Geometry: final body of the model. Coordinates: model frame, mm. A direction names the side the tool comes from. Give positions to 0.01 mm unless a question says otherwise; leave off trailing zeros. Write each loop counter-clockwise with the first axis right and the second up, starting at its lowest first coordinate (ties: lowest second). Pieces come first, ordered by that corner, then holes. Notation, with made-up numbers: (42.25, 73) -> (65.25, 73) arc R9 cw to (65.25, 87) -> close; hole circle Ø3 at (24.25, 80). An arc over 180 degrees is marked (long way). Use CSV: the item, a comma, the result in double quotes. Start each with the question number.
1) Draft query along Y for faces 1 (the face through (88.026, -49.484, -7.92)), 2 (the face through (80, -47, -1.73)), 3 (the face through (5.595, 0.246, -2.268)). Return one class per face: pulls with the +Y half, pulls with the -Y half, needs draft (parallel to the pull), parting line crosses it, or undercut.
2) Section D-D (x = 95.5). Output: boundary loops of the cut face in (y, z), plus the area to 3 significant figures.
3) Section B-B (y = -16.5). Output: boundary loops of the cut face in (x, z).
4) Contact query for flat-ended pins moving along their axis: P1, Ø1.7, axis at x = 47.5, z = -8, coming from the -Y side; P2, Ø0.9, axis at x = 127.5, z = -0.5, coming from the +Y side; P3, Ø0.6, axis at x = 43.5, z = -7.5, coming from the +Y side; P4, Ø4.5, axis at x = 0, y = 0, coming from the +Z side. Output: stop coordinate, or through.
5) Set-up query: faces 4 (the face through (135.69, -104.06, -7.95)), 5 (the face through (134.696, -103.751, -2.716)), 6 (the face through (9, 0, -4)), 7 (the face through (3, -1, -4.6)). Return all of +Z, -Z, +X, -X, +Y, -Y with unobstructed straight access to the full face (end or side cutting, diameter ignored); none if empty.
6) Section A-A (x = 124.5). Output: boundary loops of the cut face in (y, z), plus the area to 3 significant figures.
7) Section C-C (x = 0). Output: boundary loops of the cut face in (y, z).
8) Material intervals for line 1 (Y direction, x = 0, z = -6.3); line 2 (Y direction, x = 0, z = -2.7); line 3 (Z direction, x = 56, y = -2.5), sorted ascending. Write a range as [from, to].
```python
from build123d import *
from build123d.topology import SkipClean

# Parameters (mm, degrees)
EXTRUDE_1_DEPTH          = 9
SKETCH_2_R               = 5.6
CUT_EXTRUDE_1_DEPTH      = 4.6
SKETCH_3_R               = 2.6
CUT_EXTRUDE_2_DEPTH      = 178.798114195
SKETCH_5_W               = 132.43986789
SKETCH_5_H               = 5.139725872
CUT_EXTRUDE_3_DEPTH      = 181.463576917
EXTRUDE_START            = -7.270147681
SKETCH_6_R               = 4.358898944
EXTRUDE_2_DEPTH          = 7.270147681
SKETCH_7_R               = 4.358898944
EXTRUDE_3_DEPTH          = 7.270147681
SKETCH_8_R               = 2.5
EXTRUDE_4_DEPTH          = 2
CUT_EXTRUDE_4_REACH      = 179.798
SKETCH_9_R               = 1.75
CUT_EXTRUDE_5_DEPTH      = 181.463576917
CUT_EXTRUDE_5_DEPTH_BACK = 181.463576917
SKETCH_12_W              = 151.43986789
SKETCH_12_H              = 9


with BuildPart() as part:
    # 草图1 → 凸台-拉伸1 (new body)
    with BuildSketch(Plane.XY):
        with BuildLine():
            Line((97.080968947, -107.358898944), (137.080968947, -107.358898944))
            ThreePointArc((137.080968947, -107.358898944), (141.43986789, -103), (137.080968947, -98.641101056))
            Line((137.080968947, -98.641101056), (100.473705575, -98.641101056))
            Line((100.473705575, -98.641101056), (75.225539013, 1.069962639))
            ThreePointArc((75.225539013, 1.069962639), (73.67732525, 3.439757187), (71, 4.358898944))
            Line((71, 4.358898944), (9, 4.358898944))
            ThreePointArc((9, 4.358898944), (-10, 0), (9, -4.358898944))
            Line((9, -4.358898944), (67.607263372, -4.358898944))
            Line((67.607263372, -4.358898944), (92.855429934, -104.069962639))
            ThreePointArc((92.855429934, -104.069962639), (94.403643697, -106.439757187), (97.080968947, -107.358898944))
        make_face()
    extrude(amount=EXTRUDE_1_DEPTH)

    # 草图2 → 切除-拉伸1 (cut)
    with BuildSketch(Plane(origin=(0, 0, 0), x_dir=(-1, 0, 0), z_dir=(0, 0, -1))):
        Circle(SKETCH_2_R)
    extrude(amount=-CUT_EXTRUDE_1_DEPTH, mode=Mode.SUBTRACT)

    # 草图3 → 切除-拉伸2 (cut, through all)
    with BuildSketch(Plane.XY.offset(9)):
        Circle(SKETCH_3_R)
    extrude(amount=-CUT_EXTRUDE_2_DEPTH, mode=Mode.SUBTRACT)

    # 草图5 → 切除-拉伸3 (cut, through all)
    with BuildSketch(Plane(origin=(0, 4.358898944, 0), x_dir=(1, 0, 0), z_dir=(0, 1, 0))):
        with Locations((75.219933945, -4.299715255)):
            Rectangle(SKETCH_5_W, SKETCH_5_H)
    extrude(amount=-CUT_EXTRUDE_3_DEPTH, mode=Mode.SUBTRACT)

    # 草图6 → 凸台-拉伸2 (add)
    with SkipClean():  # the faces are left unmerged after this step: merging them gives an invalid solid
        with BuildSketch(Plane.XY.offset(9).offset(EXTRUDE_START)):
            with Locations(Location((71, 0, 0), (0, 0, 90))):
                Circle(SKETCH_6_R)
        extrude(amount=EXTRUDE_2_DEPTH)

    # 草图7 → 凸台-拉伸3 (add)
    with SkipClean():  # the faces are left unmerged after this step: merging them gives an invalid solid
        with BuildSketch(Plane.XY.offset(9).offset(EXTRUDE_START)):
            with Locations(Location((97.080968947, -103, 0), (0, 0, 194.209390146))):
                Circle(SKETCH_7_R)
        extrude(amount=EXTRUDE_3_DEPTH)

    # 草图8 → 凸台-拉伸4 (add)
    with SkipClean():  # the faces are left unmerged after this step: merging them gives an invalid solid
        with BuildSketch(Plane.XY.offset(1.729852319)):
            with Locations(Location((137.080968947, -103, 0), (0, 0, 180))):
                Circle(SKETCH_8_R)
        extrude(amount=EXTRUDE_4_DEPTH)

    # 草图9 → 切除-拉伸4 (cut, up to next)
    with BuildSketch(Plane.XY.offset(9), mode=Mode.PRIVATE) as cut_extrude_4_sk1:
        with Locations((137.080968947, -103)):
            Circle(SKETCH_9_R)
    cut_extrude_4_tool1 = extrude(cut_extrude_4_sk1.sketch, amount=-CUT_EXTRUDE_4_REACH, mode=Mode.PRIVATE) & part.part
    add(cut_extrude_4_tool1.solids().sort_by_distance((137.080969, -103, 9))[0], mode=Mode.SUBTRACT)

    # 镜向8: part across plane


with BuildPart() as part_1:
    add(part.part)
    add(part.part.mirror(Plane.XY))

    # 草图12 → 切除-拉伸5 (cut, two sides: drawn at the far end of the back side and taken through both)
    with BuildSketch(Plane(origin=(0, 4.358898944, 0), x_dir=(1, 0, 0), z_dir=(0, 1, 0)).offset(-CUT_EXTRUDE_5_DEPTH_BACK)):
        with Locations((65.719933945, -4.5)):
            Rectangle(SKETCH_12_W, SKETCH_12_H)
    extrude(amount=CUT_EXTRUDE_5_DEPTH + CUT_EXTRUDE_5_DEPTH_BACK, mode=Mode.SUBTRACT)


solid = part_1.part
```
Answers follow:
1,face 1,"pulls with the +Y half"
1,face 2,"needs draft"
1,face 3,"undercut"
2,outline,"(-107.06, -9) -> (-79, -9) -> (-79, -6.87) -> (-98.94, -6.87) -> (-98.94, -1.73) -> (-79, -1.73) -> (-79, 0) -> (-107.06, 0) -> close"
2,area,"150 mm^2"
3,outline,"(70.68, -9) -> (79.67, -9) -> (79.67, -6.87) -> (70.68, -6.87) -> close; (70.68, -1.73) -> (79.67, -1.73) -> (79.67, 0) -> (70.68, 0) -> close"
4,P1,"stops at y = -4.36"
4,P2,"stops at y = -98.64"
4,P3,"stops at y = 4.36"
4,P4,"passes through"
5,face 4,"-Z"
5,face 5,"none"
5,face 6,"+Y, -Y"
5,face 7,"+Z"
6,outline,"(-107.36, -9) -> (-98.64, -9) -> (-98.64, -6.87) -> (-107.36, -6.87) -> close; (-107.36, -1.73) -> (-98.64, -1.73) -> (-98.64, 0) -> (-107.36, 0) -> close"
6,area,"33.7 mm^2"
7,outline,"(-10, -9) -> (-2.6, -9) -> (-2.6, -4.6) -> (-5.6, -4.6) -> (-5.6, 0) -> (-10, 0) -> close; (2.6, -9) -> (10, -9) -> (10, 0) -> (5.6, 0) -> (5.6, -4.6) -> (2.6, -4.6) -> close"
8,line 1,"y = [-10, -2.6], [2.6, 10]"
8,line 2,"y = [-10, -5.6], [5.6, 10]"
8,line 3,"z = [-9, -6.87], [-1.73, 0]"
